Input: part model. Units: mm. Frame: model coordinates. A direction names the side the tool comes from. Give positions to 0.01 mm unless a question says otherwise; leave off trailing zeros. Loops run counter-clockwise (first coordinate to the right, second up) from the corner with the lowest first, then second, coordinate; pieces in that order, holes last. Notation, with made-up numbers: (62.25, -21) -> (68.25, -21) arc R11 cw to (68.25, -17) -> close; hole circle Ø10 at (-8, 7.25). An arc over 180 degrees is marked (long way). Answer as a JSON object with one key per item and string values.
Autodesk Inventor part; units mm, degrees
ref_plane "YZ Plane" through (0, 0, 0) normal (1, 0, 0) x (0, 1, 0)
ref_plane "XZ Plane" through (0, 0, 0) normal (0, 1, 0) x (-1, 0, 0)
ref_plane "XY Plane" through (0, 0, 0) normal (0, 0, 1) x (1, 0, 0)
sketch "Sketch1" plane through (0, 0, 0) normal (0, 1, 0) x (-1, 0, 0)
  line L0 (25, -18) -> (-25, -18)
  line L1 (-25, -18) -> (-25, 18)
  line L2 (-25, 18) -> (25, 18)
  line L3 (25, 18) -> (25, -18)
  line L4 (25, 0) -> (25, 18)
  line L5 (25, 18) -> (0, 18)
  circle A0 centre (20, 13) radius 1.75
  circle A1 centre (-20, 13) radius 1.75
  circle A2 centre (20, -13) radius 1.75
  circle A3 centre (-20, -13) radius 1.75
  line L6 (0, -18) -> (0, 18) construction
  circle A4 centre (1.27, 15.5) radius 0.5
  circle A5 centre (3.81, 15.5) radius 0.5
  circle A6 centre (-1.27, 15.5) radius 0.5
  circle A7 centre (-3.81, 15.5) radius 0.5
  circle A8 centre (-4, -13) radius 0.5
  circle A9 centre (-8, -13) radius 0.5
  circle A10 centre (4, -13) radius 0.5
  circle A11 centre (8, -13) radius 0.5
  point P0 (0, 0)
  dimension "d0" = 50
  dimension "d1" = 36
  dimension "d10" = 3.5
  dimension "d12" = 5
  dimension "d13" = 5
  dimension "d16" = 1
  dimension "d17" = 1.27
  dimension "d18" = 2.5
  dimension "d19" = 1
  dimension "d20" = 2.54
  dimension "d21" = 1
  dimension "d22" = 4
  dimension "d23" = 1
  dimension "d24" = 4
  dimension "d41" = 12
  dimension "d43" = 40
  dimension "d44" = 26
extrude "Extrusion1" add sketch "Sketch1" along normal mid plane 1.7
sketch "Sketch2" plane through (0, 0.85, 0) normal (0, 1, 0) x (1, 0, 0)
  line L0 (-14.7399, 7.1996) -> (-1.7399, 7.1996)
  line L1 (-1.7399, 7.1996) -> (-1.7399, -5.8004)
  line L2 (-1.7399, -5.8004) -> (-14.7399, -5.8004)
  line L3 (-14.7399, -5.8004) -> (-14.7399, 7.1996)
  point P0 (0, 0)
  dimension "d27" = 13
  dimension "d28" = 13
extrude "Extrusion2" add sketch "Sketch2" along normal blind 12
sketch "Sketch3" plane through (0, -0.85, 0) normal (0, -1, 0) x (1, 0, 0)
  line L0 (-14.7399, 5.8004) -> (-7.7399, 5.8004)
  line L1 (-7.7399, 5.8004) -> (-7.7399, 0.8004)
  line L2 (-7.7399, 0.8004) -> (-14.7399, 0.8004)
  line L3 (-14.7399, 0.8004) -> (-14.7399, 5.8004)
  point P0 (0, 0)
  dimension "d31" = 7
  dimension "d32" = 5
extrude "Extrusion3" add sketch "Sketch3" along normal blind 2.5
sketch "Sketch4" plane through (0, 0.85, 0) normal (0, 1, 0) x (1, 0, 0)
  line L0 (-4.7519, -12.75) -> (-3.9944, -12.75) construction
  line L1 (-3.9944, -12.75) -> (-3.9944, -13.9894) construction
  line L2 (-3.9944, -13.9894) -> (-4.7519, -13.9894) construction
  line L3 (-4.7519, -13.9894) -> (-4.7519, -12.75) construction
  line L4 (-2.1513, -12.7634) -> (-1.6525, -12.7634) construction
  line L5 (-1.6525, -12.7634) -> (-1.6525, -14.0027) construction
  line L6 (-1.6525, -14.0027) -> (-2.1513, -14.0027) construction
  line L7 (-2.1513, -14.0027) -> (-2.1513, -12.7634) construction
  line L8 (0.0686, -14.1363) -> (0.0686, -12.897) construction
  line L9 (0.0686, -12.897) -> (0.5673, -12.897) construction
  line L10 (0.5673, -12.897) -> (0.5673, -14.1363) construction
  line L11 (0.5673, -14.1363) -> (0.0686, -14.1363) construction
  line L12 (1.0686, 4.3486) -> (9.004, 4.3486) construction
  line L13 (9.004, 4.3486) -> (9.004, 3.8499) construction
  line L14 (9.004, 3.8499) -> (1.0686, 3.8499) construction
  line L15 (1.0686, 3.8499) -> (1.0686, 4.3486) construction
  line L16 (2.9588, -14.8877) -> (2.9588, -13.6483) construction
  line L17 (2.9588, -13.6483) -> (3.4575, -13.6483) construction
  line L18 (3.4575, -13.6483) -> (3.4575, -14.8877) construction
  line L19 (3.4575, -14.8877) -> (2.9588, -14.8877) construction
  line L20 (-3.0733, 9.8872) -> (-3.8308, 9.8872) construction
  line L21 (-3.8308, 9.8872) -> (-3.8308, 11.1266) construction
  line L22 (-3.8308, 11.1266) -> (-3.0733, 11.1266) construction
  line L23 (-3.0733, 11.1266) -> (-3.0733, 9.8872) construction
  line L24 (4.9547, 10.9292) -> (4.9547, 9.7419) construction
  line L25 (4.9547, 9.7419) -> (4.1972, 9.7419) construction
  line L26 (4.1972, 9.7419) -> (4.1972, 10.9292) construction
  line L27 (4.1972, 10.9292) -> (4.9547, 10.9292) construction
  line L28 (9.0783, 10.888) -> (9.0783, 9.7007) construction
  line L29 (9.0783, 9.7007) -> (8.3208, 9.7007) construction
  line L30 (8.3208, 9.7007) -> (8.3208, 10.888) construction
  line L31 (8.3208, 10.888) -> (9.0783, 10.888) construction
  line L32 (-6.789, 11.003) -> (-6.789, 9.8157) construction
  line L33 (-6.789, 9.8157) -> (-7.5465, 9.8157) construction
  line L34 (-7.5465, 9.8157) -> (-7.5465, 11.003) construction
  line L35 (-7.5465, 11.003) -> (-6.789, 11.003) construction
  point P0 (0, 0)
  point P1 (19.4358, -0.4507)
sketch "Sketch5" plane through (0, 0.85, 0) normal (0, 1, 0) x (1, 0, 0)
  circle A0 centre (-20, 13) radius 1.75
  circle A1 centre (20, 13) radius 1.75
  circle A2 centre (20, -13) radius 1.75
  circle A3 centre (-20, -13) radius 1.75
  circle A4 centre (-20, 13) radius 2.5
  circle A5 centre (-20, -13) radius 2.5
  circle A6 centre (20, 13) radius 2.5
  circle A7 centre (20, -13) radius 2.5
  point P0 (0, 0)
  dimension "d35" = 5
  dimension "d36" = 5
  dimension "d37" = 5
  dimension "d38" = 5
extrude "Extrusion4" add sketch "Sketch5" along normal blind 0.1
sketch "Sketch6" plane through (0, -0.85, 0) normal (0, -1, 0) x (1, 0, 0)
  line L0 (-3.0976, -15.0106) -> (-3.0976, -16.25) construction
  line L1 (-3.0976, -16.25) -> (-3.8551, -16.25) construction
  line L2 (-3.8551, -16.25) -> (-3.8551, -15.0106) construction
  line L3 (-3.8551, -15.0106) -> (-3.0976, -15.0106) construction
  line L4 (4.9305, -15.208) -> (4.9305, -16.3953) construction
  line L5 (4.9305, -16.3953) -> (4.173, -16.3953) construction
  line L6 (4.173, -16.3953) -> (4.173, -15.208) construction
  line L7 (4.173, -15.208) -> (4.9305, -15.208) construction
  line L8 (9.0541, -15.2492) -> (9.0541, -16.4365) construction
  line L9 (9.0541, -16.4365) -> (8.2966, -16.4365) construction
  line L10 (8.2966, -16.4365) -> (8.2966, -15.2492) construction
  line L11 (8.2966, -15.2492) -> (9.0541, -15.2492) construction
  line L12 (-6.8133, -15.1342) -> (-6.8133, -16.3215) construction
  line L13 (-6.8133, -16.3215) -> (-7.5708, -16.3215) construction
  line L14 (-7.5708, -16.3215) -> (-7.5708, -15.1342) construction
  line L15 (-7.5708, -15.1342) -> (-6.8133, -15.1342) construction
  line L16 (-4.6604, 14.3064) -> (-3.9029, 14.3064) construction
  line L17 (-3.9029, 14.3064) -> (-3.9029, 13.067) construction
  line L18 (-3.9029, 13.067) -> (-4.6604, 13.067) construction
  line L19 (-4.6604, 13.067) -> (-4.6604, 14.3064) construction
  line L20 (-2.0597, 13.0536) -> (-2.0597, 14.293) construction
  line L21 (-2.0597, 14.293) -> (-1.561, 14.293) construction
  line L22 (-1.561, 14.293) -> (-1.561, 13.0536) construction
  line L23 (-1.561, 13.0536) -> (-2.0597, 13.0536) construction
  line L24 (0.1602, 12.92) -> (0.1602, 14.1594) construction
  line L25 (0.1602, 14.1594) -> (0.6589, 14.1594) construction
  line L26 (0.6589, 14.1594) -> (0.6589, 12.92) construction
  line L27 (0.6589, 12.92) -> (0.1602, 12.92) construction
  line L28 (3.0504, 12.1687) -> (3.0504, 13.408) construction
  line L29 (3.0504, 13.408) -> (3.5491, 13.408) construction
  line L30 (3.5491, 13.408) -> (3.5491, 12.1687) construction
  line L31 (3.5491, 12.1687) -> (3.0504, 12.1687) construction
  point P0 (0, 0)
  point P1 (19.4358, -0.4507)
properties part number "UVTRON"
Q1. Section C-C, the plane z = 2. Return the cut outline in (x, y).
Evaluation:
{"outline": "(-25, -0.85) -> (-14.74, -0.85) -> (-14.74, -3.35) -> (-7.74, -3.35) -> (-7.74, -0.85) -> (25, -0.85) -> (25, 0.85) -> (-1.74, 0.85) -> (-1.74, 12.85) -> (-14.74, 12.85) -> (-14.74, 0.85) -> (-25, 0.85) -> close"}
Q2. Section D-D, the plane y = 10. Return the cut outline in (x, z), then the cut area to 3 significant figures.
Evaluation:
{"outline": "(-14.74, -7.2) -> (-1.74, -7.2) -> (-1.74, 5.8) -> (-14.74, 5.8) -> close", "area": "169 mm2"}
Q3. Ray query, line 1 along Z through (x, y) = (20, -0.5); line 2 along X through (y, z) = (0.15, 13); line 3 along X through (y, z) = (0, 12). Return the intervals inside material, ascending.
Evaluation:
{"line 1": "z = -18 to -14.75, -11.25 to 11.25, 14.75 to 18", "line 2": "x = -25 to -21.75, -18.25 to 18.25, 21.75 to 25", "line 3": "x = -25 to -21.44, -18.56 to 18.56, 21.44 to 25"}
Q4. Access query for faces 1 (the flat face through (0, 0.85, 0)), 2 (the flat face through (-7.74, -2, 3)), 3 (the flat face through (-8, 7, -7.2)), 4 (the flat face through (18, 0.95, -12)), 5 (the flat face through (-11, -2, 5.8)). Directions: +Z, -Z, +X, -X, +Y, -Y. A direction counts if a zero-diameter tool reaches every point of the face in a straight line with its end or side. Return the directions, or none.
Evaluation:
{"face 1": "+Y", "face 2": "+Z, -Z, +X, -Y", "face 3": "-Z, +X, -X, +Y", "face 4": "+Z, -Z, +X, -X, +Y", "face 5": "+Z, +X, -X, -Y"}
Q5. Draft query along X for faces 6 (the flat face through (-14.74, 7, -1)), 7 (the flat face through (-22, 0.95, -12)), 8 (the cylindrical face through (3.875, -0.012, 15.004)). Return one class per face: +X half, -X half, draft (parallel to the pull), parting line (faces both ways), or undercut.
Evaluation:
{"face 6": "-X half", "face 7": "draft", "face 8": "undercut"}
Q6. Pin query (flat end, axial travel): pin 1 (1.2 mm diameter, centred on x = -11.5, y = -2, fed in from +Z); pin 2 (3 mm diameter, centred on x = -20, z = -13, fed in from -Y); pin 3 (1 mm diameter, centred on x = -19.5, z = -6, fed in from +Y); pin 4 (1 mm diameter, centred on x = -15, y = 10.5, fed in from -Z). Return the tip coordinate at first contact, or that it passes through.
Evaluation:
{"pin 1": "stops at z = 5.8", "pin 2": "passes through", "pin 3": "stops at y = 0.85", "pin 4": "stops at z = -7.2"}
Q7. Section A-A, the plane z = 12. Return the cut outline in (x, y).
Evaluation:
{"outline": "(-25, -0.85) -> (-21.44, -0.85) -> (-21.44, 0.95) -> (-22.29, 0.95) -> (-22.29, 0.85) -> (-25, 0.85) -> close; (-18.56, -0.85) -> (18.56, -0.85) -> (18.56, 0.95) -> (17.71, 0.95) -> (17.71, 0.85) -> (-17.71, 0.85) -> (-17.71, 0.95) -> (-18.56, 0.95) -> close; (21.44, -0.85) -> (25, -0.85) -> (25, 0.85) -> (22.29, 0.85) -> (22.29, 0.95) -> (21.44, 0.95) -> close"}
